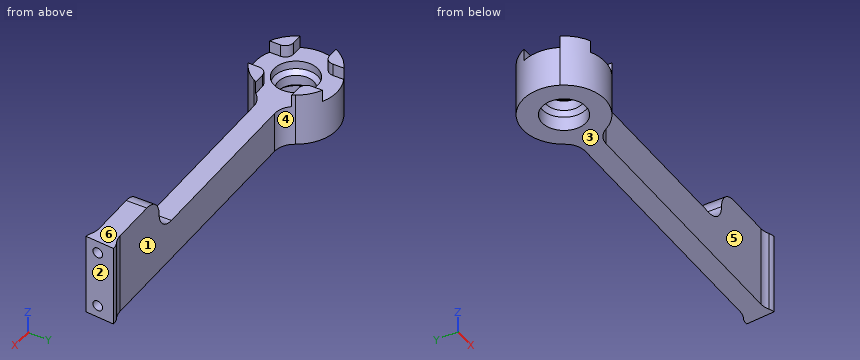
```python
from build123d import *

# Parameters (mm, degrees)
F0_R         = 5.35
F1_DEPTH     = 10
F2_START     = 3.5
F0_R_2       = 4.35
F2_DEPTH     = 4.5
F3_SIZE      = 0.99999
F4_DEPTH     = 13
F5_DEPTH     = 20
F6_R         = 1.25
F7_DEPTH     = 7.5
F8_T1_DEPTH  = 20
F8_T3_DEPTH  = 5
F8_T8_DEPTH  = 10
F8_T13_DEPTH = 10
F8_T18_DEPTH = 18.2698067281
F8_T25_DEPTH = 10
F8_T30_DEPTH = 10
F8_T35_DEPTH = 18.2698067281
F8_T39_DEPTH = 30


# Not quite as in the source:
# - a fillet or chamfer that OpenCascade refuses, or shapes differently, is made with other operations: its cross-section is extruded or revolved along the edge and cut away or added
# - a fillet or chamfer is up to 0.001 mm smaller than in the source, because OpenCascade refuses the exact size


with BuildPart() as f1:
    # F0 (on Top) → F1 (new body)
    with BuildSketch(Plane.XY):
        with BuildLine():
            Line((-4.35, 6.35), (-4.35, 9.0043045262))
            ThreePointArc((-4.35, 9.0043045262), (-7.0710678119, 7.0710678119), (-9.0043045262, 4.35))
            Line((-9.0043045262, 4.35), (-6.35, 4.35))
            ThreePointArc((-6.35, 4.35), (-4.9357864376, 4.9357864376), (-4.35, 6.35))
        make_face()
        with BuildLine():
            ThreePointArc((9.6824583655, -2.5), (9.9202969627, -1.2600429248), (10, 0))
            ThreePointArc((10, 0), (9.9202969627, 1.2600429248), (9.6824583655, 2.5))
            ThreePointArc((9.6824583655, 2.5), (9.3890575588, 3.4417434764), (9.0043045262, 4.35))
            Line((9.0043045262, 4.35), (6.35, 4.35))
            ThreePointArc((6.35, 4.35), (4.9357864376, 4.9357864376), (4.35, 6.35))
            Line((4.35, 6.35), (4.35, 9.0043045262))
            ThreePointArc((4.35, 9.0043045262), (0, 10), (-4.35, 9.0043045262))
            Line((-4.35, 9.0043045262), (-4.35, 6.35))
            ThreePointArc((-4.35, 6.35), (-4.9357864376, 4.9357864376), (-6.35, 4.35))
            Line((-6.35, 4.35), (-9.0043045262, 4.35))
            ThreePointArc((-9.0043045262, 4.35), (-10, 0), (-9.0043045262, -4.35))
            Line((-9.0043045262, -4.35), (-6.35, -4.35))
            ThreePointArc((-6.35, -4.35), (-4.9357864376, -4.9357864376), (-4.35, -6.35))
            Line((-4.35, -6.35), (-4.35, -9.0043045262))
            ThreePointArc((-4.35, -9.0043045262), (0, -10), (4.35, -9.0043045262))
            Line((4.35, -9.0043045262), (4.35, -6.35))
            ThreePointArc((4.35, -6.35), (4.9357864376, -4.9357864376), (6.35, -4.35))
            Line((6.35, -4.35), (9.0043045262, -4.35))
            ThreePointArc((9.0043045262, -4.35), (9.3890575588, -3.4417434764), (9.6824583655, -2.5))
        make_face()
        Circle(F0_R, mode=Mode.SUBTRACT)
        with BuildLine():
            ThreePointArc((-9.0043045262, -4.35), (-7.0710678119, -7.0710678119), (-4.35, -9.0043045262))
            Line((-4.35, -9.0043045262), (-4.35, -6.35))
            ThreePointArc((-4.35, -6.35), (-4.9357864376, -4.9357864376), (-6.35, -4.35))
            Line((-6.35, -4.35), (-9.0043045262, -4.35))
        make_face()
        with BuildLine():
            ThreePointArc((4.35, -9.0043045262), (7.0710678119, -7.0710678119), (9.0043045262, -4.35))
            Line((9.0043045262, -4.35), (6.35, -4.35))
            ThreePointArc((6.35, -4.35), (4.9357864376, -4.9357864376), (4.35, -6.35))
            Line((4.35, -6.35), (4.35, -9.0043045262))
        make_face()
        with BuildLine():
            Line((6.35, 4.35), (9.0043045262, 4.35))
            ThreePointArc((9.0043045262, 4.35), (7.0710678119, 7.0710678119), (4.35, 9.0043045262))
            Line((4.35, 9.0043045262), (4.35, 6.35))
            ThreePointArc((4.35, 6.35), (4.9357864376, 4.9357864376), (6.35, 4.35))
        make_face()
        with BuildLine():
            ThreePointArc((9.6824583655, 2.5), (9.9202969627, 1.2600429248), (10, 0))
            ThreePointArc((10, 0), (9.9202969627, -1.2600429248), (9.6824583655, -2.5))
            Line((9.6824583655, -2.5), (60, -2.5))
            Line((60, -2.5), (60, 2.5))
            Line((60, 2.5), (9.6824583655, 2.5))
        make_face()
        with BuildLine():
            Line((77.5505102572, 2.5), (60, 2.5))
            Line((60, 2.5), (60, -2.5))
            Line((60, -2.5), (77.5505102572, -2.5))
            ThreePointArc((77.5505102572, -2.5), (76.5, 0), (77.5505102572, 2.5))
        make_face()
        with BuildLine():
            ThreePointArc((80.3050450996, 3.4866814433), (78.8197263984, 3.2949892603), (77.5505102572, 2.5))
            ThreePointArc((77.5505102572, 2.5), (76.5, 0), (77.5505102572, -2.5))
            ThreePointArc((77.5505102572, -2.5), (78.5370404595, -3.179583209), (79.6949549004, -3.4866814433))
            Line((79.6949549004, -3.4866814433), (80, 0))
            Line((80, 0), (80.3050450996, 3.4866814433))
        make_face()
    extrude(amount=F1_DEPTH)

    # F0 (on Top) → F2 (join)
    with BuildSketch(Plane.XY.offset(F2_START)):
        Circle(F0_R)
        Circle(F0_R_2, mode=Mode.SUBTRACT)
    extrude(amount=F2_DEPTH)

    # F3 (size 1 in the source; OpenCascade refuses exactly that, so slightly less here)
    f3_edges = [f1.edges().sort_by_distance(p)[0] for p in [
        (-4.35, 0, 3.5),
        (-4.35, 0, 8),
    ]]
    chamfer(f3_edges, length=F3_SIZE)

    # F0 (on Top) → F4 (join)
    with BuildSketch(Plane.XY):
        with BuildLine():
            ThreePointArc((-9.0043045262, -4.35), (-7.0710678119, -7.0710678119), (-4.35, -9.0043045262))
            Line((-4.35, -9.0043045262), (-4.35, -6.35))
            ThreePointArc((-4.35, -6.35), (-4.9357864376, -4.9357864376), (-6.35, -4.35))
            Line((-6.35, -4.35), (-9.0043045262, -4.35))
        make_face()
        with BuildLine():
            ThreePointArc((4.35, -9.0043045262), (7.0710678119, -7.0710678119), (9.0043045262, -4.35))
            Line((9.0043045262, -4.35), (6.35, -4.35))
            ThreePointArc((6.35, -4.35), (4.9357864376, -4.9357864376), (4.35, -6.35))
            Line((4.35, -6.35), (4.35, -9.0043045262))
        make_face()
        with BuildLine():
            Line((6.35, 4.35), (9.0043045262, 4.35))
            ThreePointArc((9.0043045262, 4.35), (7.0710678119, 7.0710678119), (4.35, 9.0043045262))
            Line((4.35, 9.0043045262), (4.35, 6.35))
            ThreePointArc((4.35, 6.35), (4.9357864376, 4.9357864376), (6.35, 4.35))
        make_face()
        with BuildLine():
            Line((-4.35, 6.35), (-4.35, 9.0043045262))
            ThreePointArc((-4.35, 9.0043045262), (-7.0710678119, 7.0710678119), (-9.0043045262, 4.35))
            Line((-9.0043045262, 4.35), (-6.35, 4.35))
            ThreePointArc((-6.35, 4.35), (-4.9357864376, 4.9357864376), (-4.35, 6.35))
        make_face()
    extrude(amount=F4_DEPTH)

    # F0 (on Top) → F5 (join)
    with BuildSketch(Plane.XY):
        with BuildLine():
            ThreePointArc((80.3050450996, 3.4866814433), (78.8197263984, 3.2949892603), (77.5505102572, 2.5))
            ThreePointArc((77.5505102572, 2.5), (76.5, 0), (77.5505102572, -2.5))
            ThreePointArc((77.5505102572, -2.5), (78.5370404595, -3.179583209), (79.6949549004, -3.4866814433))
            Line((79.6949549004, -3.4866814433), (80, 0))
            Line((80, 0), (80.3050450996, 3.4866814433))
        make_face()
        with BuildLine():
            Line((77.5505102572, 2.5), (60, 2.5))
            Line((60, 2.5), (60, -2.5))
            Line((60, -2.5), (77.5505102572, -2.5))
            ThreePointArc((77.5505102572, -2.5), (76.5, 0), (77.5505102572, 2.5))
        make_face()
    extrude(amount=F5_DEPTH)

    # F6 (on face) → F7 (cut)
    with BuildSketch(Plane(origin=(79.3923101205, -6.9459271067, 0), x_dir=(0.0871557427, 0.9961946981, 0), z_dir=(0.9961946981, -0.0871557427, 0))):
        with Locations((6.4724594198, 17)):
            Circle(F6_R)
        with Locations((6.4724594198, 3)):
            Circle(F6_R)
    extrude(amount=-F7_DEPTH, mode=Mode.SUBTRACT)

    # F8: fillet of radius 5 on 6 edges, made by hand

    # F8_s2 → F8_t1 (join)
    with BuildSketch(Plane.XY):
        with BuildLine():
            ThreePointArc((78.3529411765, 3.0882352941), (77.2126781252, 2.6492874993), (76, 2.5))
            Line((76, 2.5), (77.5505102572, 2.5))
            ThreePointArc((77.5505102572, 2.5), (77.9307168562, 2.822776518), (78.3529411765, 3.0882352941))
        make_face()
        with BuildLine():
            ThreePointArc((76, -2.5), (77.2126781252, -2.6492874993), (78.3529411765, -3.0882352941))
            ThreePointArc((78.3529411765, -3.0882352941), (77.9307168562, -2.822776518), (77.5505102572, -2.5))
            Line((77.5505102572, -2.5), (76, -2.5))
        make_face()
    extrude(amount=F8_T1_DEPTH)

    # F8_s4 → F8_t3 (join)
    with BuildSketch(Plane.XZ.offset(-2.5)):
        with BuildLine():
            ThreePointArc((55, 10), (58.5355339059, 11.4644660941), (60, 15))
            Line((60, 15), (60, 10))
            Line((60, 10), (55, 10))
        make_face()
    extrude(amount=F8_T3_DEPTH)


with BuildPart() as f8_tool6:
    # F8_s7 → F8_t8 (new body)
    with BuildSketch(Plane.XY):
        with BuildLine():
            ThreePointArc((8.6602540378, 5), (10.4903810568, 3.1698729811), (12.9903810568, 2.5))
            Line((12.9903810568, 2.5), (9.6824583655, 2.5))
            ThreePointArc((9.6824583655, 2.5), (9.2561479341, 3.7846697903), (8.6602540378, 5))
        make_face()
    extrude(amount=F8_T8_DEPTH)

    split(bisect_by=Plane.XZ.offset(-4.35), keep=Keep.BOTTOM)


with BuildPart() as f1_1:
    add(f1.part)

    # F8_t5: union F8_tool6
    add(f8_tool6.part)


with BuildPart() as f8_tool11:
    # F8_s12 → F8_t13 (new body)
    with BuildSketch(Plane.XY):
        with BuildLine():
            ThreePointArc((8.6602540378, 5), (10.4903810568, 3.1698729811), (12.9903810568, 2.5))
            Line((12.9903810568, 2.5), (9.6824583655, 2.5))
            ThreePointArc((9.6824583655, 2.5), (9.2561479341, 3.7846697903), (8.6602540378, 5))
        make_face()
    extrude(amount=F8_T13_DEPTH)

    split(bisect_by=Plane.XZ.offset(-4.35), keep=Keep.TOP)


with BuildPart() as f1_2:
    add(f1_1.part)

    # F8_t10: union F8_tool11
    add(f8_tool11.part)


with BuildPart() as f8_tool16:
    # F8_s17 → F8_t18 (new body)
    with BuildSketch(Plane.XY):
        with BuildLine():
            ThreePointArc((8.6602540378, 5), (10.4903810568, 3.1698729811), (12.9903810568, 2.5))
            Line((12.9903810568, 2.5), (9.6824583655, 2.5))
            ThreePointArc((9.6824583655, 2.5), (9.2561479341, 3.7846697903), (8.6602540378, 5))
        make_face()
    extrude(amount=F8_T18_DEPTH)

    split(bisect_by=Plane.XY.offset(10), keep=Keep.TOP)

    split(bisect_by=Plane.XZ.offset(-4.35), keep=Keep.BOTTOM)

    split(bisect_by=Plane.XY.offset(13), keep=Keep.BOTTOM)


with BuildPart() as f1_3:
    add(f1_2.part)

    # F8_t15: union F8_tool16
    add(f8_tool16.part)


with BuildPart() as f8_tool23:
    # F8_s24 → F8_t25 (new body)
    with BuildSketch(Plane.XY):
        with BuildLine():
            ThreePointArc((8.6602540378, -5), (10.4903810568, -3.1698729811), (12.9903810568, -2.5))
            Line((12.9903810568, -2.5), (9.6824583655, -2.5))
            ThreePointArc((9.6824583655, -2.5), (9.2561479341, -3.7846697903), (8.6602540378, -5))
        make_face()
    extrude(amount=F8_T25_DEPTH)

    split(bisect_by=Plane.XZ.offset(4.35), keep=Keep.TOP)


with BuildPart() as f1_4:
    add(f1_3.part)

    # F8_t22: union F8_tool23
    add(f8_tool23.part)


with BuildPart() as f8_tool28:
    # F8_s29 → F8_t30 (new body)
    with BuildSketch(Plane.XY):
        with BuildLine():
            ThreePointArc((8.6602540378, -5), (10.4903810568, -3.1698729811), (12.9903810568, -2.5))
            Line((12.9903810568, -2.5), (9.6824583655, -2.5))
            ThreePointArc((9.6824583655, -2.5), (9.2561479341, -3.7846697903), (8.6602540378, -5))
        make_face()
    extrude(amount=F8_T30_DEPTH)

    split(bisect_by=Plane.XZ.offset(4.35), keep=Keep.BOTTOM)


with BuildPart() as f1_5:
    add(f1_4.part)

    # F8_t27: union F8_tool28
    add(f8_tool28.part)


with BuildPart() as f8_tool33:
    # F8_s34 → F8_t35 (new body)
    with BuildSketch(Plane.XY):
        with BuildLine():
            ThreePointArc((8.6602540378, -5), (10.4903810568, -3.1698729811), (12.9903810568, -2.5))
            Line((12.9903810568, -2.5), (9.6824583655, -2.5))
            ThreePointArc((9.6824583655, -2.5), (9.2561479341, -3.7846697903), (8.6602540378, -5))
        make_face()
    extrude(amount=F8_T35_DEPTH)

    split(bisect_by=Plane.XY.offset(10), keep=Keep.TOP)

    split(bisect_by=Plane.XY.offset(13), keep=Keep.BOTTOM)

    split(bisect_by=Plane.XZ.offset(4.35), keep=Keep.TOP)


with BuildPart() as f1_6:
    add(f1_5.part)

    # F8_t32: union F8_tool33
    add(f8_tool33.part)

    # F8_s40 → F8_t39 (cut)
    with BuildSketch(Plane.XZ.offset(-15)):
        with BuildLine():
            ThreePointArc((60, 15), (61.4644660941, 18.5355339059), (65, 20))
            Line((65, 20), (60, 20))
            Line((60, 20), (60, 15))
        make_face()
    extrude(amount=F8_T39_DEPTH, mode=Mode.SUBTRACT)


solid = f1_6.part
```
Geometry: final body of the model. Coordinates: model frame, mm. Face numbers are marked on the shaded views. A direction names the side the tool comes from. Coordinates: 2 decimals unless noted, no trailing zeros. Order: outer loops, then holes, each group sorted by start corner. A loop starts at its lowest first (then second) coordinate and runs counter-clockwise, first axis right, second up. Notation, with made-up numbers: (32.5, 70.25) -> (63.5, 70.25) arc R30 cw to (63.5, 98.25) -> close; hole circle Ø1 at (-19.5, 19.5). An arc over 180 degrees is marked (long way). Write each question's results on one line, items separated by ' | '. Start each with the question number.
1) Material intervals for line 1 along Y through (x, z) = (0, 5.9); line 2 along Y through (x, z) = (0, 9.45); line 3 along Y through (x, z) = (51, 3.75), sorted ascending.
2) First-contact query: pin 1 (1.5 mm diameter, centred on x = 26, y = 1.5, fed in from +Z); pin 2 (1.3 mm diameter, centred on x = -8, z = 11.5, fed in from -Y); pin 3 (11.5 mm diameter, centred on x = 0, y = 0, fed in from -Z); pin 4 (0.8 mm diameter, centred on x = -7.5, z = 11, fed in from +Y). Flat tips, straight axial feed; report the tip coordinate or a pass-through.
3) Cut plane C-C, the plane x = 21. Output: boundary loops of the cut face in (y, z), and give its area (3 significant figures).
4) Cut plane B-B, the plane x = 59. Output: boundary loops of the cut face in (y, z), and give its area (3 significant figures).
5) Mould query, pull axis X, two halves, no side actions, for the marked faces 1, 2 and 3. Classes: released by +X, released by -X, zero draft, split by the parting line, or undercut.
6) Set-up query: the marked faces 4, 5 and 6. Return all of +Z, -Z, +X, -X, +Y, -Y with unobstructed straight access to the full face (end or side cutting, diameter ignored); none if empty.
Checks:
1) line 1: -10 to -4.35, 4.35 to 10 | line 2: -10 to -5.35, 5.35 to 10 | line 3: -2.5 to 2.5
2) pin 1: z = 10 | pin 2: y = -6.78 | pin 3: z = 0 | pin 4: y = 7.04
3) outline: (-2.5, 0) -> (2.5, 0) -> (2.5, 10) -> (-2.5, 10) -> close | area: 50.0 mm^2
4) outline: (-2.5, 0) -> (2.5, 0) -> (2.5, 12) -> (-2.5, 12) -> close | area: 60.0 mm^2
5) face 1: undercut | face 2: released by +X | face 3: zero draft
6) face 4: +Z, -Z, +Y | face 5: +Z, -Z, -Y | face 6: +Z, +X, -X, +Y, -Y
